Could you check a few things on this model? Use its own coordinates, in mm. Face numbers are marked on the shaded views. A direction names the side the tool comes from. Give positions to 0.01 mm unless a question says otherwise; leave off trailing zeros. Loops run counter-clockwise (first coordinate to the right, second up) from the corner with the lowest first, then second, coordinate; pieces in that order, holes last. Notation, with made-up numbers: M 5,45.25 L 45,45.25 A4 cw 45,52.25 Z; hole C 56,60.25 d3. An arc over 180 degrees is marked long. Use CSV: the item, a comma, the result in double quotes.
```python
from build123d import *

# Parameters (mm, degrees)
IZIM1_R                     = 80
Y_KSEKLIK_EKSTR_ZYON1_DEPTH = 26
IZIM1_7_R                   = 80
IZIM1_7_R_2                 = 75
Y_KSEKLIK_EKSTR_ZYON2_DEPTH = 160
IZIM1_9_R                   = 75
IZIM1_9_R_2                 = 70
Y_KSEKLIK_EKSTR_ZYON3_DEPTH = 146


with BuildPart() as part:
    # izim1 → Y_kseklik-Ekstr_zyon1 (new body)
    with BuildSketch(Plane(origin=(0, 0, 0), x_dir=(1, 0, 0), z_dir=(0, 1, 0))):
        with BuildLine():
            Line((108.086576189, 65.169734496), (108.086576189, -129.830265504))
            ThreePointArc((108.086576189, -129.830265504), (115.157644, -146.901333316), (98.086576189, -139.830265504))
            Line((98.086576189, -139.830265504), (-96.913423811, -139.830265504))
            ThreePointArc((-96.913423811, -139.830265504), (-113.984491623, -146.901333316), (-106.913423811, -129.830265504))
            Line((-106.913423811, -129.830265504), (-106.913423811, 65.169734496))
            ThreePointArc((-106.913423811, 65.169734496), (-113.984491623, 82.240802308), (-96.913423811, 75.169734496))
            Line((-96.913423811, 75.169734496), (98.086576189, 75.169734496))
            ThreePointArc((98.086576189, 75.169734496), (115.157644, 82.240802308), (108.086576189, 65.169734496))
        make_face()
        with Locations((0.586576189, -32.330265504)):
            Circle(IZIM1_R, mode=Mode.SUBTRACT)
    extrude(amount=Y_KSEKLIK_EKSTR_ZYON1_DEPTH)

    # izim1_7 → Y_kseklik-Ekstr_zyon2 (add)
    with BuildSketch(Plane(origin=(0, 0, 0), x_dir=(1, 0, 0), z_dir=(0, 1, 0))):
        with Locations((0.586576189, -32.330265504)):
            Circle(IZIM1_7_R)
        with Locations((0.586576189, -32.330265504)):
            Circle(IZIM1_7_R_2, mode=Mode.SUBTRACT)
    extrude(amount=Y_KSEKLIK_EKSTR_ZYON2_DEPTH)

    # izim1_9 → Y_kseklik-Ekstr_zyon3 (add)
    with BuildSketch(Plane(origin=(0, 0, 0), x_dir=(1, 0, 0), z_dir=(0, 1, 0))):
        with Locations((0.586576189, -32.330265504)):
            Circle(IZIM1_9_R)
        with Locations((0.586576189, -32.330265504)):
            Circle(IZIM1_9_R_2, mode=Mode.SUBTRACT)
    extrude(amount=Y_KSEKLIK_EKSTR_ZYON3_DEPTH)


solid = part.part
```
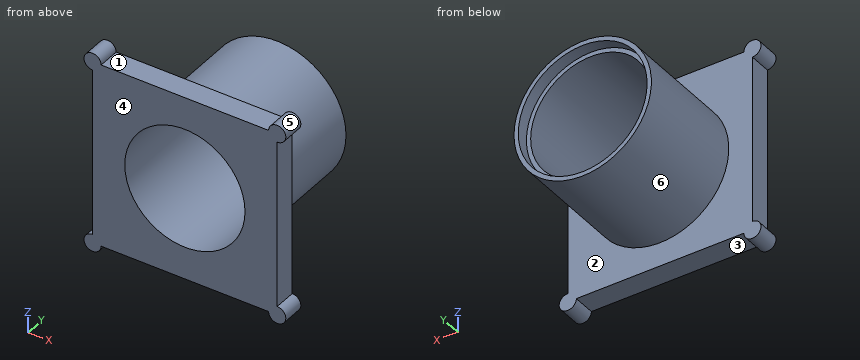
1. I want a section at B-B, the plane x = -10.5. List the corners of the cut face in (y, z) for me, then the cut area to 3 significant figures.
Outcome:
outline,"M 0,-75.17 L 26,-75.17 L 26,-46.9 L 160,-46.9 L 160,-41.85 L 146,-41.85 L 146,-36.79 L 0,-36.79 Z; M 0,101.45 L 146,101.45 L 146,106.51 L 160,106.51 L 160,111.56 L 26,111.56 L 26,139.83 L 0,139.83 Z"
area,"4,560 mm2"
2. If we mould it in two halves opening along Z, with no side actions, what happens to the marked faces 4, 5 and 6? For each: +Z half, -Z half, draft (parallel to the pull), parting line (faces both ways), or undercut.
Outcome:
face 4,"draft"
face 5,"undercut"
face 6,"parting line"
3. I want a section at A-A, the plane z = 52. List the corners of the cut face in (x, y) for me.
Outcome:
outline,"M -106.91,0 L -66.59,0 L -66.59,146 L -71.79,146 L -71.79,160 L -76.96,160 L -76.96,26 L -106.91,26 Z; M 67.77,0 L 108.09,0 L 108.09,26 L 78.13,26 L 78.13,160 L 72.96,160 L 72.96,146 L 67.77,146 Z"
4. I want a section at D-D, the plane x = -89. List the corners of the cut face in (y, z) for me, then the cut area to 3 significant figures.
Outcome:
outline,"M 0,-75.17 L 26,-75.17 L 26,139.83 L 0,139.83 Z"
area,"5,590 mm2"
5. I'm going to push flat-ended pins straight in: pin 1 Ø13 at (x, y) = (34, 14.5) entering from -Z; pin 2 Ø5 at (y, z) = (121, -18.5) entering from +X; pin 3 Ø12 at (x, z) = (-50, -6) entering from -Y; pin 4 Ø5 at (x, z) = (87, 86.5) entering from +Y. Where does each tip first touch, or does it pass through?
Outcome:
pin 1,"z = -75.17"
pin 2,"x = 64.34"
pin 3,"through"
pin 4,"y = 26"
6. I want a section at C-C, the plane y = 12. List the corners of the cut face in (x, z) for me, then the cut area to 3 significant figures.
Outcome:
outline,"M -106.91,-65.17 A10 ccw long -96.91,-75.17 L 98.09,-75.17 A10 ccw long 108.09,-65.17 L 108.09,129.83 A10 ccw long 98.09,139.83 L -96.91,139.83 A10 ccw long -106.91,129.83 Z; hole C 0.59,32.33 d140"
area,"31,800 mm2"
7. Please list where these lines run through material, in increasing order: line 1 (Y direction, x = -11, z = -49); line 2 (Z direction, x = -73.5, y = 14); line 3 (X direction, y = 131.5, z = 75.5).
Outcome:
line 1,"0 to 26"
line 2,"-75.17 to 139.83"
line 3,"-66.77 to -54.52, 55.69 to 67.94"
8. Which directions (+Z, -Z, +X, -X, +Y, -Y) give clear straight access to the entire face, cutting with the end or side of a thin tool? Please do the marked faces 1, 2 and 3.
Outcome:
face 1,"+Z, +Y, -Y"
face 2,"+Y"
face 3,"-Z, +Y, -Y"
